Build history of the part. All positions in model axes, mm. Face numbers are marked on the shaded views. Coordinates: 2 decimals unless noted, no trailing zeros. Loops run counter-clockwise (first coordinate to the right, second up) from the corner with the lowest first, then second, coordinate; pieces in that order, holes last.
(1) Flat gauge pins, fed straight in: P1, Ø12, axis at y = 6, z = 43.5, coming from the +X side; P2, Ø2, axis at y = -7.5, z = 45, coming from the -X side; P3, Ø9, axis at x = -16.5, y = 9.52, coming from the +Z side; P4, Ø3, axis at x = -24.5, z = 43.5, coming from the -Y side. Where does each tip first touch, or does it go through?
(2) Wall check: L1, parallel to Y at x = 0, z = 34 (3 decimals); L2, parallel to Y at x = 13, z = 42; L3, parallel to Y at x = -18.5, z = 17.5. Give the ranges that are in metal, low to high.
(3) Slice it at C-C (z = 47.5). Give the number of separate pieces and of enclosed holes in the cut face, and give its area (3 significant figures).
(4) Slice it at B-B (x = -16). Give the cut face in (y, z), and give its area (3 significant figures).
(5) Two-plate mould, pull along X, no slides. Class the marked faces 1, 2 and 3: pulls with the +X half, pulls with the -X half, needs draft (parallel to the pull), parting line crosses it, or undercut.
(6) Slice it at A-A (y = -19.05). Give the cut face in (x, z) (3 decimals).
(7) Slice it at D-D (x = 14). Give the cut face in (y, z), and give its area (3 significant figures).
from build123d import *

# Parameters (mm, degrees)
F0_R     = 31.75
F0_R_2   = 5.715
F1_DEPTH = 50.8
F3_DEPTH = 76.2
F4_R     = 3.175
F5_DEPTH = 76.2


with BuildPart() as f1:
    # F0 (on Top) → F1 (new body)
    with BuildSketch(Plane.XY):
        Circle(F0_R)
        with Locations((-16.4977839421, -9.525)):
            Circle(F0_R_2, mode=Mode.SUBTRACT)
        with Locations((0, -19.05)):
            Circle(F0_R_2, mode=Mode.SUBTRACT)
        with Locations((16.4977839421, -9.525)):
            Circle(F0_R_2, mode=Mode.SUBTRACT)
        with Locations((-16.4977839421, 9.525)):
            Circle(F0_R_2, mode=Mode.SUBTRACT)
        with Locations((16.4977839421, 9.525)):
            Circle(F0_R_2, mode=Mode.SUBTRACT)
        with BuildLine():
            ThreePointArc((0, 13.335), (-4.0411152545, 23.0911152545), (5.715, 19.05))
            ThreePointArc((5.715, 19.05), (4.0411152545, 15.0088847455), (0, 13.335))
        make_face(mode=Mode.SUBTRACT)
    extrude(amount=F1_DEPTH)

    # F2 (on face) → F3 (cut)
    with BuildSketch(Plane.XY.offset(50.8)):
        with BuildLine():
            ThreePointArc((21.7238685359, 27.4185818051), (17.2514556231, 32.9968613186), (10.8342089276, 29.8443029222))
            ThreePointArc((10.8342089276, 29.8443029222), (16.0088685359, 27.4185818051), (20.6648408036, 24.1044986374))
            ThreePointArc((20.6648408036, 24.1044986374), (21.4526772444, 25.6789922716), (21.7238685359, 27.4185818051))
        make_face()
        with BuildLine():
            ThreePointArc((20.6648408036, 24.1044986374), (16.0088685359, 27.4185818051), (10.8342089276, 29.8443029222))
            ThreePointArc((10.8342089276, 29.8443029222), (13.1272721994, 22.4832370801), (20.6648408036, 24.1044986374))
        make_face()
        with BuildLine():
            Line((-15.740754111, 27.5733777405), (-12.907418371, 22.6101697472))
            ThreePointArc((-12.907418371, 22.6101697472), (-10.798399472, 24.7038210459), (-10.025754111, 27.5733777405))
            ThreePointArc((-10.025754111, 27.5733777405), (-10.1564827093, 28.7887533666), (-10.5426877637, 29.9485264198))
            ThreePointArc((-10.5426877637, 29.9485264198), (-13.1952704408, 28.8781463739), (-15.740754111, 27.5733777405))
        make_face()
        with BuildLine():
            ThreePointArc((-18.6103108055, 22.6310231015), (-15.7616515985, 21.8584159475), (-12.907418371, 22.6101697472))
            Line((-12.907418371, 22.6101697472), (-15.740754111, 27.5733777405))
            Line((-15.740754111, 27.5733777405), (-18.6103108055, 22.6310231015))
        make_face()
        with BuildLine():
            Line((-18.6103108055, 22.6310231015), (-15.740754111, 27.5733777405))
            ThreePointArc((-15.740754111, 27.5733777405), (-18.1584784341, 26.0448106339), (-20.4288200251, 24.3048516223))
            ThreePointArc((-20.4288200251, 24.3048516223), (-19.6111339829, 23.368453883), (-18.6103108055, 22.6310231015))
        make_face()
        with BuildLine():
            Line((-31.75, 0), (-26.0367194254, 0))
            ThreePointArc((-26.0367194254, 0), (-26.0351468655, 0.0773908676), (-26.0346226469, 0.1547959354))
            ThreePointArc((-26.0346226469, 0.1547959354), (-26.7776126488, 2.9726571064), (-28.8133948529, 5.0578349259))
            Line((-28.8133948529, 5.0578349259), (-31.75, 0))
        make_face()
        with BuildLine():
            ThreePointArc((-31.2630289527, -5.5394512999), (-27.5927222778, -3.7671174142), (-26.0367194254, 0))
            Line((-26.0367194254, 0), (-31.75, 0))
            ThreePointArc((-31.75, 0), (-31.6280229326, -2.7804074119), (-31.2630289527, -5.5394512999))
        make_face()
        with BuildLine():
            ThreePointArc((-31.2075285673, 5.8440277824), (-31.614091257, 2.9345756072), (-31.75, 0))
            Line((-31.75, 0), (-28.8133948529, 5.0578349259))
            ThreePointArc((-28.8133948529, 5.0578349259), (-29.9665899591, 5.5845306834), (-31.2075285673, 5.8440277824))
        make_face()
        with BuildLine():
            ThreePointArc((-10.2938685359, -27.4185818051), (-14.2692790024, -21.9747730965), (-20.6648408036, -24.1044986374))
            ThreePointArc((-20.6648408036, -24.1044986374), (-16.0088685359, -27.4185818051), (-10.8342089276, -29.8443029222))
            ThreePointArc((-10.8342089276, -29.8443029222), (-10.4305890224, -28.6611688923), (-10.2938685359, -27.4185818051))
        make_face()
        with BuildLine():
            ThreePointArc((20.4288200251, -24.3048516223), (12.907418371, -22.6101697472), (10.5426877637, -29.9485264198))
            ThreePointArc((10.5426877637, -29.9485264198), (15.740754111, -27.5733777405), (20.4288200251, -24.3048516223))
        make_face()
        with BuildLine():
            ThreePointArc((31.75, 0), (31.6280229326, 2.7804074119), (31.2630289527, 5.5394512999))
            ThreePointArc((31.2630289527, 5.5394512999), (26.0346905704, -0.126932667), (31.2075285673, -5.8440277824))
            ThreePointArc((31.2075285673, -5.8440277824), (31.614091257, -2.9345756072), (31.75, 0))
        make_face()
    extrude(amount=-F3_DEPTH, mode=Mode.SUBTRACT)

    # F4 (on face) → F5 (cut)
    with BuildSketch(Plane.XY.offset(50.8)):
        Circle(F4_R)
    extrude(amount=-F5_DEPTH, mode=Mode.SUBTRACT)


solid = f1.part
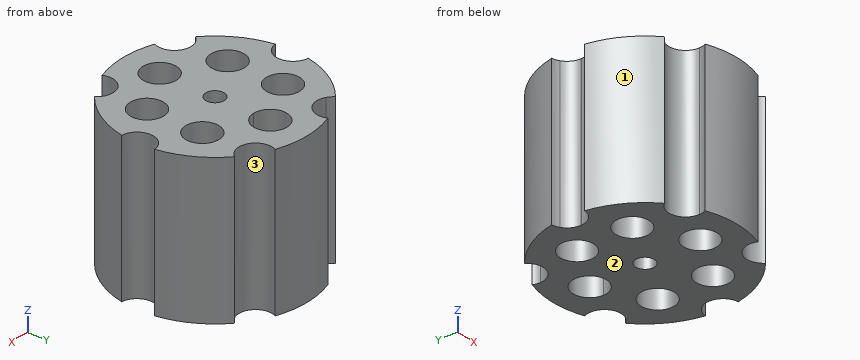
Response values:
1. P1: stops at x = 31.26
1. P2: stops at x = -31.08
1. P3: passes through
1. P4: stops at y = -21.89
2. L1: y = -31.75 to -24.765, -13.335 to -3.175, 3.175 to 13.335, 24.765 to 31.75
2. L2: y = -22.56 to -14.04, -5.01 to 5.01, 14.04 to 22.56
2. L3: y = -22.28 to -14.88, -4.17 to 4.17, 14.88 to 22.57
3. separate pieces: 1
3. enclosed holes: 7
3. area: 2,220 mm2
4. outline: (-21.7, 0) - (-15.22, 0) - (-15.22, 50.8) - (-21.7, 50.8) - close; (-3.83, 0) - (3.83, 0) - (3.83, 50.8) - (-3.83, 50.8) - close; (15.22, 0) - (21.86, 0) - (21.86, 50.8) - (15.22, 50.8) - close
4. area: 1,060 mm2
5. face 1: pulls with the -X half
5. face 2: needs draft
5. face 3: undercut
6. outline: (-25.4, 0) - (-5.715, 0) - (-5.715, 50.8) - (-25.4, 50.8) - close; (5.715, 0) - (25.4, 0) - (25.4, 50.8) - (5.715, 50.8) - close
7. outline: (-22.13, 0) - (-14.67, 0) - (-14.67, 50.8) - (-22.13, 50.8) - close; (-4.38, 0) - (4.38, 0) - (4.38, 50.8) - (-4.38, 50.8) - close; (14.67, 0) - (22.07, 0) - (22.07, 50.8) - (14.67, 50.8) - close
7. area: 1,200 mm2
